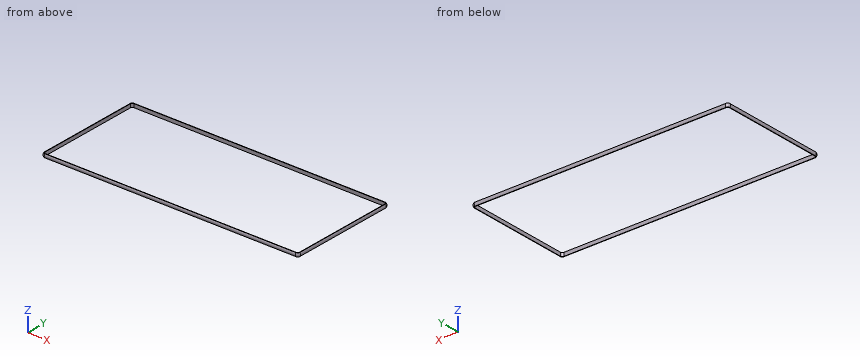
from build123d import *

# Parameters (mm, degrees)
F1_DEPTH = 25.4
F2_W     = 1804.67
F2_H     = 25.4
F3_DEPTH = 6.35
F5_DEPTH = 2540


with BuildPart() as f1:
    # F0 (on Top) → F1 (new body)
    with BuildSketch(Plane.XY):
        with BuildLine():
            ThreePointArc((917.575, 368.935), (913.1113073453, 379.7113073453), (902.335, 384.175))
            Line((902.335, 384.175), (-902.335, 384.175))
            ThreePointArc((-902.335, 384.175), (-913.1113073453, 379.7113073453), (-917.575, 368.935))
            Line((-917.575, 368.935), (-917.575, -368.935))
            ThreePointArc((-917.575, -368.935), (-913.1113073453, -379.7113073453), (-902.335, -384.175))
            Line((-902.335, -384.175), (902.335, -384.175))
            ThreePointArc((902.335, -384.175), (913.1113073453, -379.7113073453), (917.575, -368.935))
            Line((917.575, -368.935), (917.575, 368.935))
        make_face()
        with BuildLine():
            ThreePointArc((914.4, -368.3), (910.6802561211, -377.2802561211), (901.7, -381))
            Line((901.7, -381), (-901.7, -381))
            ThreePointArc((-901.7, -381), (-910.6802561211, -377.2802561211), (-914.4, -368.3))
            Line((-914.4, -368.3), (-914.4, 368.3))
            ThreePointArc((-914.4, 368.3), (-910.6802561211, 377.2802561211), (-901.7, 381))
            Line((-901.7, 381), (901.7, 381))
            ThreePointArc((901.7, 381), (910.6802561211, 377.2802561211), (914.4, 368.3))
            Line((914.4, 368.3), (914.4, -368.3))
        make_face(mode=Mode.SUBTRACT)
    extrude(amount=F1_DEPTH)

    # F2 (on face) → F3 (join)
    with BuildSketch(Plane.XZ.offset(384.175)):
        with Locations((0, 12.7)):
            Rectangle(F2_W, F2_H)
    extrude(amount=F3_DEPTH)

    # F4 (on face) → F5 (cut)
    with BuildSketch(Plane(origin=(-902.335, 0, 0), x_dir=(0, -1, 0), z_dir=(-1, 0, 0))):
        with BuildLine():
            ThreePointArc((384.175, 25.4), (388.7056210694, 12.7), (384.175, 0))
            Line((384.175, 0), (390.525, 0))
            Line((390.525, 0), (390.525, 25.4))
            Line((390.525, 25.4), (384.175, 25.4))
        make_face()
    extrude(amount=-F5_DEPTH, mode=Mode.SUBTRACT)

    # F6: sweep along a path in F6_path
    with BuildLine(Plane(origin=(-902.335, -384.175, 25.4), x_dir=(0, 1, 0), z_dir=(0, 0, 1))) as f6_path:
        ThreePointArc((0, 0), (4.4636926547, 10.7763073453), (15.24, 15.24))
        Line((15.24, 15.24), (753.11, 15.24))
        ThreePointArc((753.11, 15.24), (763.8863073453, 10.7763073453), (768.35, 0))
        Line((768.35, 0), (768.35, -1804.67))
        ThreePointArc((768.35, -1804.67), (763.8863073453, -1815.4463073453), (753.11, -1819.91))
        Line((753.11, -1819.91), (15.24, -1819.91))
        ThreePointArc((15.24, -1819.91), (4.4636926547, -1815.4463073453), (0, -1804.67))
        Line((0, -1804.67), (0, 0))
    # F3_face (on face) → F6 (sweep)
    with BuildSketch(Plane(origin=(-902.335, -387.35, 12.7), x_dir=(0, -1, 0), z_dir=(-1, 0, 0))):
        with BuildLine():
            Line((-3.175, 12.7), (-3.175, -12.7))
            ThreePointArc((-3.175, -12.7), (1.3556210694, 0), (-3.175, 12.7))
        make_face()
    sweep(path=f6_path.line)


solid = f1.part
The listing builds one solid part. Answer for the finished solid, in the listing's coordinates (mm). Give positions to 0.01 mm unless a question says otherwise; leave off trailing zeros. Write each loop counter-clockwise with the first axis right and the second up, starting at its lowest first coordinate (ties: lowest second). Pieces come first, ordered by that corner, then holes.
Item 1: Section A-A, the plane y = 145 is taken. Write down the section's boundary in (x, z) (3 decimals).
Item 2: Flat-ended cylindrical pins translate along their axes: P1, Ø1, axis at y = 250, z = 3, coming from the -X side; P2, Ø4, axis at x = 190, z = 19.5, coming from the -Y side; P3, Ø10, axis at y = 168, z = 20, coming from the +X side. Find the tip coordinate at first contact, or state that the pin passes through.
Item 3: Section B-B, the plane x = 51 is taken. Write down the section's boundary in (y, z) (3 decimals), plus the area to 3 significant figures.
Item 4: Find the intervals of material crossed by line 1 along Y through (x, z) = (-272, 9.75); line 2 along X through (y, z) = (-190.5, 16); line 3 along X through (y, z) = (184.5, 16.5), in increasing order.
Completed:
1. outline: (-917.575, 0) - (-914.4, 0) - (-914.4, 25.4) - (-917.575, 25.4) arc R20.065 ccw to start; (914.4, 0) - (917.575, 0) arc R20.065 ccw to (917.575, 25.4) - (914.4, 25.4) - close
2. P1: stops at x = -919.87
2. P2: stops at y = -388.12
2. P3: stops at x = 921.97
3. outline: (-384.175, 0) - (-381, 0) - (-381, 25.4) - (-384.175, 25.4) arc R20.065 ccw to start; (381, 0) - (384.175, 0) arc R20.065 ccw to (384.175, 25.4) - (381, 25.4) - close
3. area: 319 mm2
4. line 1: y = -388.49 to -381, 381 to 388.49
4. line 2: x = -921.83 to -914.4, 914.4 to 921.83
4. line 3: x = -921.74 to -914.4, 914.4 to 921.74
